CAD build for the part. Positions are in the model's coordinates, mm. A direction names the side the tool comes from. Coordinates: 2 decimals unless noted, no trailing zeros. Order: outer loops, then holes, each group sorted by start corner. A loop starts at its lowest first (then second) coordinate and runs counter-clockwise, first axis right, second up. Notation, with made-up numbers: (85, -23) - (95, -23) arc R17 ccw to (95, -19) - close; hole circle Ø7 at (-35, 33.25). An arc over 180 degrees is marked (long way). Write each question's results on one line, items separated by ' | '. Start each with the question number.
Q1. Band-saw the part on B-B, the plane z = 15. Write the cut outline in (x, y) (3 decimals).
Q2. Which spindle directions (+Z, -Z, +X, -X, +Y, -Y) get a long thin tool onto all of the face, cutting with end or side? Do faces 4 (the cylindrical face through (-17.82, -1.485, -6.188)), 5 (the flat face through (-24.311, -1, -25)), 6 (the flat face through (-1, -3.175, 8)), 7 (the cylindrical face through (-11.716, -1.485, -36.896)). Say none if no direction does.
Q3. Wall check: probe 1 along X at (y, z) = (-3, 4.5); probe 2 along X at (y, z) = (-0.5, 14.5); probe 3 along X at (y, z) = (-0.55, -25.5). Give the ranges that are in metal, low to high.
Q4. Pull direction X, two halves, no side cores. Call faces 1 (the cylindrical face through (-0.171, -1.485, -39.903)), 2 (the flat face through (-11.611, -1, -27)), 3 (the cylindrical face through (11.723, -1.485, -36.928)): released by +X, released by -X, zero draft, split by the parting line, or undercut.
Q5. Pin check, flat tips, straight feed: P1, Ø2, axis at x = -13.5, y = -2.5, coming from the -Z side; P2, Ø1, axis at y = -2.5, z = -1, coming from the +X side; P3, Ø1, axis at y = -1.5, z = -24, coming from the +X side; P4, Ø8, axis at x = -21, z = -21, coming from the -Y side (3 decimals). Stop position of each tip, or through.
Q6. Band-saw the part on C-C, the plane y = -0.75. Count the separate pieces of the cut face and the enclosed holes in it, then the cut area to 3 significant figures.
Q7. Band-saw the part on A-A, the plane x = 0. Write the cut outline in (y, z) (3 decimals).
Q8. Band-saw the part on D-D, the plane x = -13. Write the cut outline in (y, z) (3 decimals), then the cut area to 3 significant figures.
```python
from build123d import *

# Parameters (mm, degrees)
BOSS_EXTRUDE1_DEPTH      = 3.175
BOSS_EXTRUDE1_DEPTH_BACK = 0.254
BOSS_EXTRUDE2_DEPTH      = 3.429
LPATTERN1_COUNT          = 8
LPATTERN1_PITCH          = 2.45
FILLET1_R                = 0.3


with BuildPart() as part:
    # Sketch3 → Boss-Extrude1 (new body, two sides)
    with BuildSketch(Plane.XZ) as boss_extrude1_sk:
        with BuildLine():
            ThreePointArc((39.9034, 0), (-17.63815803, 35.793528925), (-24.310512242, -31.643013859))
            Line((-24.310512242, -31.643013859), (-24.310512242, -17.960512242))
            ThreePointArc((-24.310512242, -17.960512242), (-17.960512242, -11.610512242), (-11.610512242, -17.960512242))
            Line((-11.610512242, -17.960512242), (-11.610512242, -35.740512242))
            ThreePointArc((-11.610512242, -35.740512242), (-11.71946636, -36.911770666), (-12.042589815, -38.042835884))
            ThreePointArc((-12.042589815, -38.042835884), (0, -39.9034), (12.042589815, -38.042835884))
            ThreePointArc((12.042589815, -38.042835884), (11.71946636, -36.911770666), (11.610512242, -35.740512242))
            Line((11.610512242, -35.740512242), (11.610512242, -17.960512242))
            ThreePointArc((11.610512242, -17.960512242), (17.960512242, -11.610512242), (24.310512242, -17.960512242))
            Line((24.310512242, -17.960512242), (24.310512242, -31.643013859))
            ThreePointArc((24.310512242, -31.643013859), (35.793528925, -17.63815803), (39.9034, 0))
        make_face()
        with BuildLine():
            ThreePointArc((-5.55625, 0), (0, 5.55625), (5.55625, 0))
            Line((5.55625, 0), (5.55625, -17.78))
            ThreePointArc((5.55625, -17.78), (0, -23.33625), (-5.55625, -17.78))
            Line((-5.55625, -17.78), (-5.55625, 0))
        make_face(mode=Mode.SUBTRACT)
        with BuildLine():
            ThreePointArc((-11.590512242, 0.180512242), (-17.960512242, -6.189487758), (-24.330512242, 0.180512242))
            Line((-24.330512242, 0.180512242), (-24.330512242, 17.960512242))
            ThreePointArc((-24.330512242, 17.960512242), (-17.960512242, 24.330512242), (-11.590512242, 17.960512242))
            Line((-11.590512242, 17.960512242), (-11.590512242, 0.180512242))
        make_face(mode=Mode.SUBTRACT)
        with BuildLine():
            ThreePointArc((24.310512242, 0.180512242), (17.960512242, -6.169487758), (11.610512242, 0.180512242))
            Line((11.610512242, 0.180512242), (11.610512242, 17.960512242))
            ThreePointArc((11.610512242, 17.960512242), (17.960512242, 24.310512242), (24.310512242, 17.960512242))
            Line((24.310512242, 17.960512242), (24.310512242, 0.180512242))
        make_face(mode=Mode.SUBTRACT)
    extrude(amount=BOSS_EXTRUDE1_DEPTH)
    extrude(boss_extrude1_sk.sketch, amount=-BOSS_EXTRUDE1_DEPTH_BACK)

    # Sketch4 → Boss-Extrude2 (add)
    with BuildSketch(Plane(origin=(0, 0.254, 0), x_dir=(1, 0, 0), z_dir=(0, 1, 0))):
        Polygon((-5.55625, -0.803750085), (-3.69625, -0.34), (-3.69625, 0.34), (-5.55625, 0.803750085), align=None)
    boss_extrude2 = extrude(amount=-BOSS_EXTRUDE2_DEPTH)

    # LPattern1: Boss-Extrude2 ×8
    with Locations(*[(0, 0, -i * LPATTERN1_PITCH) for i in range(1, LPATTERN1_COUNT)]):
        add(boss_extrude2)

    # Fillet1
    fillet1_edges = [part.edges().sort_by_distance(p)[0] for p in [
        (-3.69625, -1.4605, 0.34),
        (-5.55625, -1.4605, -0.803750085),
        (-3.69625, -1.4605, -0.34),
        (-5.499846219, -1.4605, 0.789687043),
        (-5.55625, -1.4605, -1.646249915),
        (-5.55625, -1.4605, -3.253750085),
        (-3.69625, -1.4605, -2.79),
        (-3.69625, -1.4605, -2.11),
        (-5.55625, -1.4605, -4.096249915),
        (-5.55625, -1.4605, -5.703750085),
        (-3.69625, -1.4605, -5.24),
        (-3.69625, -1.4605, -4.56),
        (-5.55625, -1.4605, -6.546249915),
        (-5.55625, -1.4605, -8.153750085),
        (-3.69625, -1.4605, -7.69),
        (-3.69625, -1.4605, -7.01),
        (-5.55625, -1.4605, -8.996249915),
        (-5.55625, -1.4605, -10.603750085),
        (-3.69625, -1.4605, -10.14),
        (-3.69625, -1.4605, -9.46),
        (-5.55625, -1.4605, -11.446249915),
        (-5.55625, -1.4605, -13.053750085),
        (-3.69625, -1.4605, -12.59),
        (-3.69625, -1.4605, -11.91),
        (-5.55625, -1.4605, -13.896249915),
        (-5.55625, -1.4605, -15.503750085),
        (-3.69625, -1.4605, -15.04),
        (-3.69625, -1.4605, -14.36),
        (-5.55625, -1.4605, -16.346249915),
        (-3.69625, -1.4605, -17.49),
        (-3.69625, -1.4605, -16.81),
    ]]
    fillet(fillet1_edges, radius=FILLET1_R)


solid = part.part
```
Results below:
1) outline: (-36.977, -3.175) - (-24.331, -3.175) - (-24.331, 0.254) - (-36.977, 0.254) - close; (-11.591, -3.175) - (11.611, -3.175) - (11.611, 0.254) - (-11.591, 0.254) - close; (24.311, -3.175) - (36.977, -3.175) - (36.977, 0.254) - (24.311, 0.254) - close
2) face 4: +Y, -Y | face 5: -Z, +Y, -Y | face 6: +Z, -Z, +X, -X, -Y | face 7: -X, +Y, -Y
3) probe 1: x = -39.65 to -24.33, -11.59 to -3.26, 3.26 to 11.61, 24.31 to 39.65 | probe 2: x = -37.18 to -24.33, -11.59 to 11.61, 24.31 to 37.18 | probe 3: x = -30.69 to -24.31, -11.61 to 11.61, 24.31 to 30.69
4) face 1: split by the parting line | face 2: undercut | face 3: released by +X
5) P1: stops at z = -14.72 | P2: stops at x = 39.9 | P3: stops at x = 32.25 | P4: stops at y = -3.175
6) separate pieces: 1 | enclosed holes: 3 | area: 3,450 mm²
7) outline: (-3.175, -39.903) - (0.254, -39.903) - (0.254, -23.336) - (-3.175, -23.336) - close; (-3.175, 5.556) - (0.254, 5.556) - (0.254, 39.903) - (-3.175, 39.903) - close
8) outline: (-3.175, -13.996) - (0.254, -13.996) - (0.254, -3.816) - (-3.175, -3.816) - close; (-3.175, 21.957) - (0.254, 21.957) - (0.254, 37.726) - (-3.175, 37.726) - close | area: 89.0 mm²
